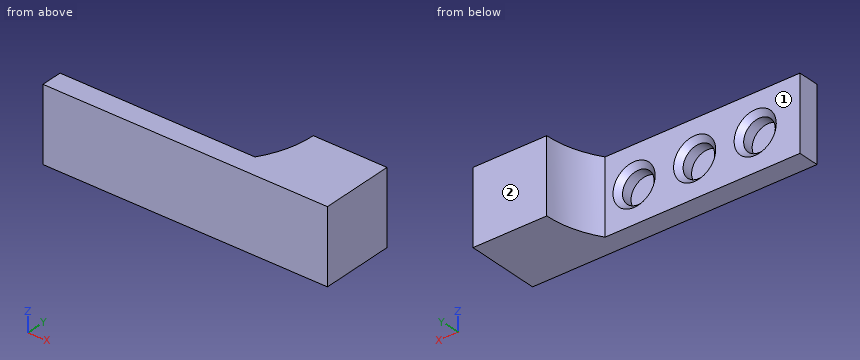
Autodesk Inventor part; units mm, degrees
ref_plane "YZ Plane" through (0, 0, 0) normal (1, 0, 0) x (0, 1, 0)
ref_plane "XZ Plane" through (0, 0, 0) normal (0, 1, 0) x (-1, 0, 0)
ref_plane "XY Plane" through (0, 0, 0) normal (0, 0, 1) x (1, 0, 0)
sketch "Sketch1" plane through (0, 0, 0) normal (0, 1, 0) x (-1, 0, 0)
  line L0 (-13.5, -3.5) -> (13.5, -3.5)
  line L1 (13.5, -3.5) -> (13.5, 3.5)
  line L2 (13.5, 3.5) -> (-13.5, 3.5)
  line L3 (-13.5, 3.5) -> (-13.5, -3.5)
  line L4 (-13.5, -3.5) -> (13.5, 3.5) construction
  line L5 (13.5, -3.5) -> (-13.5, 3.5) construction
  line L6 (-6.5, 3.5) -> (-6.5, -3.5)
  line L7 (-6.5, 0) -> (13.5, 0) construction
  circle A0 centre (9.25, 0) radius 1.5
  circle A1 centre (3.5, 0) radius 1.5
  circle A2 centre (-2.25, 0) radius 1.5
  point P0 (0, 0)
  dimension "d0" = 27
  dimension "d1" = 7
  dimension "d2" = 7
  dimension "d3" = 3
  dimension "d6" = 3
  dimension "d11" = 3
  dimension "d19" = 5.75
  dimension "d20" = 5.75
  dimension "d21" = 4.25
  dimension "d22" = 4.25
extrude "Extrusion1" add sketch "Sketch1" along normal blind 7 contours L3 L2 L6 L0
extrude "Extrusion2" add sketch "Sketch1" along normal blind 2 contours L6 L2 L1 L0
extrude "Extrusion3" add sketch "Sketch1" along normal blind 0.5 contours A0 | A1 | A2
chamfer "Chamfer1" distance 0.5 angle 45 3 edges at (3.75, 2, 0) (-2, 2, 0) (-7.75, 2, 0)
sketch "Sketch2" plane through (13.5, 7, -3.5) normal (0, 0, -1) x (-1, 0, 0)
  line L0 (0, -7) -> (27, -7)
  line L1 (27, -7) -> (27, -5)
  line L2 (7, -5) -> (27, -5)
  line L3 (7, -5) -> (7, 0)
  line L4 (0, 0) -> (7, 0)
  line L5 (0, -7) -> (0, 0)
  arc A0 (7, 0) -> (8.5, -5) centre (16.0833, 0) ccw
  point P0 (13.5, -7)
  dimension "d32" = 1.5
extrude "Extrusion4" add sketch "Sketch2" against normal up to surface (7 mm away) contours A0 L2 L3
equation "\"d20\" = d19"
equation "\"d21\" = d19 - 0.5 * d11"
equation "\"d22\" = d19 - 0.5 * d3"
properties part number "glue_test_flex"
Geometry check sheet. Reference: the model listing, model coordinates, mm. Face numbers are marked on the shaded views. A direction names the side the tool comes from. Round coordinates to 2 decimals unless told otherwise and drop trailing zeros. Order: outer loops, then holes, each group sorted by start corner. A loop starts at its lowest first (then second) coordinate and runs counter-clockwise, first axis right, second up. Notation, with made-up numbers: (71, -24.5) - (112, -24.5) arc R29 cw to (112, -4.5) - close; hole circle Ø8 at (-3, 17.25). An arc over 180 degrees is marked (long way). One line per question, with ' | ' between items. Start each with the question number.
(1) Sectioned sample at B-B on x = -9.25. Record the cut outline in (y, z), and give its area (3 significant figures).
(2) Depth check by flat-ended pin: pin 1 Ø3.5 at (x, z) = (-6, -1.5) entering from +Y; pin 2 Ø3 at (x, z) = (-6, 1.5) entering from -Y; pin 3 Ø1.5 at (x, z) = (-9, 0.5) entering from +Y; pin 4 Ø2.5 at (x, z) = (-3.5, -0.5) entering from +Y. Enter the tip coordinate at first touch or a pass-through.
(3) Thickness scan on L1, parallel to Z at x = -3.5, y = 1.2; L2, parallel to Y at x = -11.75, z = 2.75; L3, parallel to Y at x = -3.75, z = -0.25. Record the ranges inside material, lowest first. Write a range as [from, to].
(4) Sectioned sample at D-D on z = -3. Record the cut outline in (x, y), and give its area (3 significant figures).
(5) Sectioned sample at C-C on z = 0. Record the cut outline in (x, y), and give its area (3 significant figures).
(6) Sectioned sample at A-A on y = 0.75. Record the cut outline in (x, z).
(7) Access from +Z, -Z, +X, -X, +Y, -Y to the whole of each face (thin tool, end or side, straight path). Record for the marked faces 1 and 2.
Conclusion:
1) outline: (0, -3.5) - (2, -3.5) - (2, -2) - (1.5, -1.5) - (0.5, -1.5) - (0.5, 1.5) - (1.5, 1.5) - (2, 2) - (2, 3.5) - (0, 3.5) - close | area: 9.25 mm2
2) pin 1: stops at y = 2 | pin 2: stops at y = 0 | pin 3: stops at y = 0.5 | pin 4: stops at y = 1.75
3) L1: z = [-3.5, -1.5], [1.5, 3.5] | L2: y = [0, 2] | L3: y = [0, 0.5]
4) outline: (-13.5, 0) - (13.5, 0) - (13.5, 7) - (6.5, 7) arc R9.08 cw to (5, 2) - (-13.5, 2) - close | area: 91.4 mm2
5) outline: (-13.5, 0) - (13.5, 0) - (13.5, 7) - (6.5, 7) arc R9.08 cw to (5, 2) - (4.25, 2) - (3.75, 1.5) - (3.75, 0.5) - (0.75, 0.5) - (0.75, 1.5) - (0.25, 2) - (-1.5, 2) - (-2, 1.5) - (-2, 0.5) - (-5, 0.5) - (-5, 1.5) - (-5.5, 2) - (-7.25, 2) - (-7.75, 1.5) - (-7.75, 0.5) - (-10.75, 0.5) - (-10.75, 1.5) - (-11.25, 2) - (-13.5, 2) - close | area: 77.2 mm2
6) outline: (-13.5, -3.5) - (13.5, -3.5) - (13.5, 3.5) - (-13.5, 3.5) - close; hole circle Ø3 at (-9.25, 0); hole circle Ø3 at (-3.5, 0); hole circle Ø3 at (2.25, 0)
7) face 1: +Z, -Z, -X, +Y | face 2: +Z, -Z, +X, -X, +Y
